from build123d import *

# Parameters (mm, degrees)
F0_W     = 25
F0_H     = 35
F1_DEPTH = 2
F2_R     = 3
F3_W     = 4
F3_H     = 2
F4_DEPTH = 100


with BuildPart() as f1:
    # F0 (on Top) → F1 (new body)
    with BuildSketch(Plane.XY):
        with Locations((12.5, 17.5)):
            Rectangle(F0_W, F0_H)
    extrude(amount=F1_DEPTH)

    # F2
    f2_edges = [f1.edges().sort_by_distance(p)[0] for p in [
        (25, 35, 1),
        (0, 35, 1),
        (25, 0, 1),
        (0, 0, 1),
    ]]
    fillet(f2_edges, radius=F2_R)

    # F3 (on face) → F4 (cut)
    with BuildSketch(Plane.XY.offset(2)):
        Polygon((10.5, 30), (6, 30), (6, 5), (19, 5), (19, 30), (14.5, 30), (14.5, 28), (10.5, 28), align=None)
        with Locations((12.5, 31)):
            Rectangle(F3_W, F3_H)
        with Locations((12.5, 29)):
            Rectangle(F3_W, F3_H)
    extrude(amount=-F4_DEPTH, mode=Mode.SUBTRACT)


solid = f1.part
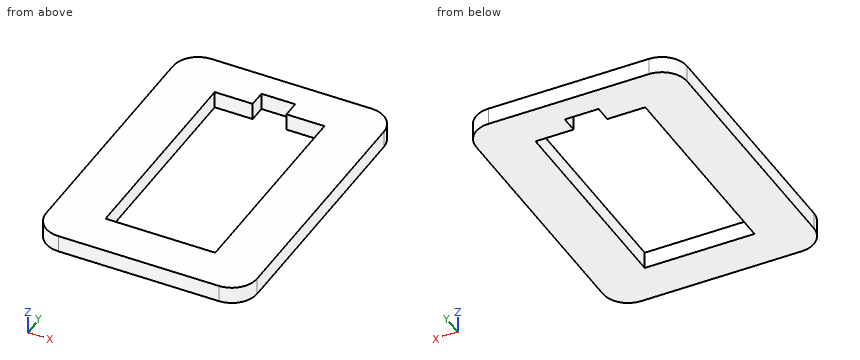
Can you work these out from the model? Positions are in its coordinate system, mm. Give positions to 0.01 mm unless a question says otherwise; leave off trailing zeros. Order: outer loops, then holes, each group sorted by start corner. A loop starts at its lowest first (then second) coordinate and runs counter-clockwise, first axis right, second up. Notation, with made-up numbers: M 59.5,7.25 L 70.5,7.25 A21 cw 70.5,18.25 Z; hole C 84,-40 d9. An arc over 180 degrees is marked long. Use one line per item in the form item = value. Start each with the question number.
Item 1: If we section it at B-B (y = 9): Write out the boundary of the cut face in (x, z), then the cut area to 3 significant figures.
Item 2: If I drill on line 1 along X through (y, z) = (20, 0.65); line 2 along Y through (x, z) = (17.5, 0.3); line 3 along Y through (x, z) = (2.75, 0.9), over which ranges is the centre line in solid material (lowest first)?
Item 3: If we section it at C-C (x = 1.5): Write out the boundary of the cut face in (y, z), then the cut area to 3 significant figures.
Item 4: If we section it at A-A (z = 0.75): Write out the boundary of the cut face in (x, y), then the cut area to 3 significant figures.
Outcome:
q1.outline = M 0,0 L 6,0 L 6,2 L 0,2 Z; M 19,0 L 25,0 L 25,2 L 19,2 Z
q1.area = 24.0 mm2
q2.line_1 = 0 to 6, 19 to 25
q2.line_2 = 0 to 5, 30 to 35
q2.line_3 = 0.01 to 34.99
q3.outline = M 0.4,0 L 34.6,0 L 34.6,2 L 0.4,2 Z
q3.area = 68.4 mm2
q4.outline = M 0,3 A3 ccw 3,0 L 22,0 A3 ccw 25,3 L 25,32 A3 ccw 22,35 L 3,35 A3 ccw 0,32 Z; hole M 6,5 L 19,5 L 19,30 L 14.5,30 L 14.5,32 L 10.5,32 L 10.5,30 L 6,30 Z
q4.area = 534 mm2
